Source: CAD feature listing. Evaluate the final solid. Frame: model axes, mm. A direction names the side the tool comes from. Coordinates: 2 decimals unless noted, no trailing zeros. Order: outer loops, then holes, each group sorted by start corner. A loop starts at its lowest first (then second) coordinate and runs counter-clockwise, first axis right, second up.
```python
from build123d import *

# Parameters (mm, degrees)
SKETCH_1_W          = 70
SKETCH_1_H          = 5
EXTRUDE_1_DEPTH     = 22
EXTRUDE_2_DEPTH     = 10
SKETCH_3_R          = 1.7
CUT_EXTRUDE_1_DEPTH = 8
SKETCH_5_R          = 1.7
CUT_EXTRUDE_2_DEPTH = 8


with BuildPart() as part:
    # 草圖1 → 填料-伸長1 (new body)
    with BuildSketch(Plane.XY):
        with Locations((2.778517987, 7.348484848)):
            Rectangle(SKETCH_1_W, SKETCH_1_H)
    extrude(amount=EXTRUDE_1_DEPTH)

    # 草圖2 → 填料-伸長2 (add)
    with BuildSketch(Plane.XY.offset(22)):
        Polygon((-32.221482013, 1.848484848), (-30.705054647, 1.848484848), (-29.90120707, 4.848484848), (-32.221482013, 4.848484848), align=None)
        Polygon((-25.84420707, 1.848484848), (-22.585054647, 1.848484848), (-21.78120707, 4.848484848), (-26.648054647, 4.848484848), align=None)
        Polygon((-18.528054647, 4.848484848), (-17.72420707, 1.848484848), (-14.465054647, 1.848484848), (-13.66120707, 4.848484848), align=None)
        Polygon((-10.408054647, 4.848484848), (-9.60420707, 1.848484848), (-6.345054647, 1.848484848), (-5.54120707, 4.848484848), align=None)
        Polygon((-2.288054647, 4.848484848), (-1.48420707, 1.848484848), (1.774945353, 1.848484848), (2.57879293, 4.848484848), align=None)
        Polygon((5.831945353, 4.848484848), (6.63579293, 1.848484848), (9.894945353, 1.848484848), (10.69879293, 4.848484848), align=None)
        Polygon((13.951945353, 4.848484848), (14.75579293, 1.848484848), (18.014945353, 1.848484848), (18.81879293, 4.848484848), align=None)
        Polygon((22.071945353, 4.848484848), (22.87579293, 1.848484848), (26.134945353, 1.848484848), (26.93879293, 4.848484848), align=None)
        Polygon((30.191945353, 4.848484848), (30.99579293, 1.848484848), (34.254945353, 1.848484848), (35.05879293, 4.848484848), align=None)
    extrude(amount=-EXTRUDE_2_DEPTH)

    # 草圖3 → 除料-伸長1 (cut)
    with BuildSketch(Plane(origin=(0, 0, 0), x_dir=(-1, 0, 0), z_dir=(0, 0, -1))):
        with Locations((-32.778517987, 7.348484848)):
            Circle(SKETCH_3_R)
        with Locations((-2.778517987, 7.348484848)):
            Circle(SKETCH_3_R)
        with Locations((27.221482013, 7.348484848)):
            Circle(SKETCH_3_R)
    extrude(amount=-CUT_EXTRUDE_1_DEPTH, mode=Mode.SUBTRACT)

    # 草圖5 → 除料-伸長2 (cut)
    with BuildSketch(Plane.ZY.offset(32.221482013)):
        with Locations((10, 7.348484848)):
            Circle(SKETCH_5_R)
        with Locations((18, 7.348484848)):
            Circle(SKETCH_5_R)
    extrude(amount=-CUT_EXTRUDE_2_DEPTH, mode=Mode.SUBTRACT)


solid = part.part
```
1. Section query C-C on y = 3.25. Count the separate pieces of the cut face and the enclosed holes in it, plus the area to 3 significant figures.
Findings:
separate pieces: 9
enclosed holes: 0
area: 340 mm2
2. Ray query, line 1 (X direction, y = 7.25, z = 7.75); line 2 (Y direction, x = -30, z = 10); line 3 (X direction, y = 8.5, z = 17.25). Return the intervals inside material, ascending.
Findings:
line 1: x = -32.22 to -28.92, -25.52 to 1.08, 4.48 to 31.08, 34.48 to 37.78
line 2: y = 4.85 to 5.65, 9.05 to 9.85
line 3: x = -24.22 to 37.78
3. Section query A-A on z = 10. Return loops of the section in (x, y).
Findings:
outline: (-32.22, 4.85) - (37.78, 4.85) - (37.78, 9.85) - (-32.22, 9.85) - (-32.22, 9.05) - (-24.22, 9.05) - (-24.22, 5.65) - (-32.22, 5.65) - close
4. Draft query along X for faces 1 (the face through (14.35, 3.37, 17.07)), 2 (the face through (2.3, 9.6, 0)), 3 (the face through (34.65, 3.33, 17.07)). Return one class per face: released by +X, released by -X, zero draft, split by the parting line, or undercut.
Findings:
face 1: undercut
face 2: zero draft
face 3: released by +X
5. Section query D-D on x = -3. Return loops of the section in (y, z), plus the area to 3 significant figures.
Findings:
outline: (4.85, 0) - (9.85, 0) - (9.85, 22) - (4.85, 22) - close
area: 110 mm2
6. Section query B-B on z = 6.25. Return loops of the section in (x, y).
Findings:
outline: (-32.22, 4.85) - (37.78, 4.85) - (37.78, 9.85) - (-32.22, 9.85) - close; hole circle Ø3.4 at (-27.22, 7.35); hole circle Ø3.4 at (2.78, 7.35); hole circle Ø3.4 at (32.78, 7.35)
7. Access query for faces 4 (the face through (-24, 3, 12)), 5 (the face through (-27, 7, 8)), 6 (the face through (-5, 4.848, 8)). Directions: +Z, -Z, +X, -X, +Y, -Y. A direction counts if a zero-diameter tool reaches every point of the face in a straight line with its end or side. Return the directions, or none.
Findings:
face 4: -Z, +X, -X, -Y
face 5: -Z
face 6: -Z, -Y
8. Pin query (flat end, axial travel): P1, Ø1, axis at y = 8, z = 18.5, coming from the -X side; P2, Ø0.9, axis at x = 16.5, y = 3, coming from the -Z side; P3, Ø3, axis at y = 3, z = 5.5, coming from the +X side; P4, Ø4, axis at x = 0.5, z = 7, coming from the -Y side. Return the tip coordinate at first contact, or that it passes through.
Findings:
P1: stops at x = -24.22
P2: stops at z = 12
P3: passes through
P4: stops at y = 4.85
